```python
from build123d import *

# Parameters (mm, degrees)
SKETCH1_R           = 2.1
BOSS_EXTRUDE1_DEPTH = 1000


with BuildPart() as part:
    # Sketch1 → Boss-Extrude1 (new body)
    with BuildSketch(Plane(origin=(0, 0, 0), x_dir=(-1, 0, 0), z_dir=(0, 0, -1))):
        with BuildLine():
            Line((15.499339828, -8.2), (12.84, -8.2))
            Line((12.84, -8.2), (14.64, -10))
            Line((14.64, -10), (25.36, -10))
            Line((25.36, -10), (27.16, -8.2))
            Line((27.16, -8.2), (24.500660172, -8.2))
            Line((24.500660172, -8.2), (24.500660172, -6.56))
            Line((24.500660172, -6.56), (27.16, -3.900660172))
            Line((27.16, -3.900660172), (32.84, -3.900660172))
            Line((32.84, -3.900660172), (35.499339828, -6.56))
            Line((35.499339828, -6.56), (35.499339828, -8.2))
            Line((35.499339828, -8.2), (32.84, -8.2))
            Line((32.84, -8.2), (34.64, -10))
            Line((34.64, -10), (38, -10))
            ThreePointArc((38, -10), (39.414213562, -9.414213562), (40, -8))
            Line((40, -8), (40, -4.64))
            Line((40, -4.64), (38.2, -2.84))
            Line((38.2, -2.84), (38.2, -5.499339828))
            Line((38.2, -5.499339828), (36.56, -5.499339828))
            Line((36.56, -5.499339828), (33.900660172, -2.84))
            Line((33.900660172, -2.84), (33.900660172, 2.84))
            Line((33.900660172, 2.84), (36.56, 5.499339828))
            Line((36.56, 5.499339828), (38.2, 5.499339828))
            Line((38.2, 5.499339828), (38.2, 2.84))
            Line((38.2, 2.84), (40, 4.64))
            Line((40, 4.64), (40, 8))
            ThreePointArc((40, 8), (39.414213562, 9.414213562), (38, 10))
            Line((38, 10), (34.64, 10))
            Line((34.64, 10), (32.84, 8.2))
            Line((32.84, 8.2), (35.499339828, 8.2))
            Line((35.499339828, 8.2), (35.499339828, 6.56))
            Line((35.499339828, 6.56), (32.84, 3.900660172))
            Line((32.84, 3.900660172), (27.16, 3.900660172))
            Line((27.16, 3.900660172), (24.500660172, 6.56))
            Line((24.500660172, 6.56), (24.500660172, 8.2))
            Line((24.500660172, 8.2), (27.16, 8.2))
            Line((27.16, 8.2), (25.36, 10))
            Line((25.36, 10), (14.64, 10))
            Line((14.64, 10), (12.84, 8.2))
            Line((12.84, 8.2), (15.499339828, 8.2))
            Line((15.499339828, 8.2), (15.499339828, 6.56))
            Line((15.499339828, 6.56), (12.84, 3.900660172))
            Line((12.84, 3.900660172), (7.16, 3.900660172))
            Line((7.16, 3.900660172), (4.500660172, 6.56))
            Line((4.500660172, 6.56), (4.500660172, 8.2))
            Line((4.500660172, 8.2), (7.16, 8.2))
            Line((7.16, 8.2), (5.36, 10))
            Line((5.36, 10), (-5.36, 10))
            Line((-5.36, 10), (-7.16, 8.2))
            Line((-7.16, 8.2), (-4.500660172, 8.2))
            Line((-4.500660172, 8.2), (-4.500660172, 6.56))
            Line((-4.500660172, 6.56), (-7.16, 3.900660172))
            Line((-7.16, 3.900660172), (-12.84, 3.900660172))
            Line((-12.84, 3.900660172), (-15.499339828, 6.56))
            Line((-15.499339828, 6.56), (-15.499339828, 8.2))
            Line((-15.499339828, 8.2), (-12.84, 8.2))
            Line((-12.84, 8.2), (-14.64, 10))
            Line((-14.64, 10), (-25.36, 10))
            Line((-25.36, 10), (-27.16, 8.2))
            Line((-27.16, 8.2), (-24.500660172, 8.2))
            Line((-24.500660172, 8.2), (-24.500660172, 6.56))
            Line((-24.500660172, 6.56), (-27.16, 3.900660172))
            Line((-27.16, 3.900660172), (-32.84, 3.900660172))
            Line((-32.84, 3.900660172), (-35.499339828, 6.56))
            Line((-35.499339828, 6.56), (-35.499339828, 8.2))
            Line((-35.499339828, 8.2), (-32.84, 8.2))
            Line((-32.84, 8.2), (-34.64, 10))
            Line((-34.64, 10), (-38, 10))
            ThreePointArc((-38, 10), (-39.414213562, 9.414213562), (-40, 8))
            Line((-40, 8), (-40, 4.64))
            Line((-40, 4.64), (-38.2, 2.84))
            Line((-38.2, 2.84), (-38.2, 5.499339828))
            Line((-38.2, 5.499339828), (-36.56, 5.499339828))
            Line((-36.56, 5.499339828), (-33.900660172, 2.84))
            Line((-33.900660172, 2.84), (-33.900660172, -2.84))
            Line((-33.900660172, -2.84), (-36.56, -5.499339828))
            Line((-36.56, -5.499339828), (-38.2, -5.499339828))
            Line((-38.2, -5.499339828), (-38.2, -2.84))
            Line((-38.2, -2.84), (-40, -4.64))
            Line((-40, -4.64), (-40, -8))
            ThreePointArc((-40, -8), (-39.414213562, -9.414213562), (-38, -10))
            Line((-38, -10), (-34.64, -10))
            Line((-34.64, -10), (-32.84, -8.2))
            Line((-32.84, -8.2), (-35.499339828, -8.2))
            Line((-35.499339828, -8.2), (-35.499339828, -6.56))
            Line((-35.499339828, -6.56), (-32.84, -3.900660172))
            Line((-32.84, -3.900660172), (-27.16, -3.900660172))
            Line((-27.16, -3.900660172), (-24.500660172, -6.56))
            Line((-24.500660172, -6.56), (-24.500660172, -8.2))
            Line((-24.500660172, -8.2), (-27.16, -8.2))
            Line((-27.16, -8.2), (-25.36, -10))
            Line((-25.36, -10), (-14.64, -10))
            Line((-14.64, -10), (-12.84, -8.2))
            Line((-12.84, -8.2), (-15.499339828, -8.2))
            Line((-15.499339828, -8.2), (-15.499339828, -6.56))
            Line((-15.499339828, -6.56), (-12.84, -3.900660172))
            Line((-12.84, -3.900660172), (-7.16, -3.900660172))
            Line((-7.16, -3.900660172), (-4.500660172, -6.56))
            Line((-4.500660172, -6.56), (-4.500660172, -8.2))
            Line((-4.500660172, -8.2), (-7.16, -8.2))
            Line((-7.16, -8.2), (-5.36, -10))
            Line((-5.36, -10), (5.36, -10))
            Line((5.36, -10), (7.16, -8.2))
            Line((7.16, -8.2), (4.500660172, -8.2))
            Line((4.500660172, -8.2), (4.500660172, -6.56))
            Line((4.500660172, -6.56), (7.16, -3.900660172))
            Line((7.16, -3.900660172), (12.84, -3.900660172))
            Line((12.84, -3.900660172), (15.499339828, -6.56))
            Line((15.499339828, -6.56), (15.499339828, -8.2))
        make_face()
        with Locations(Location((10, 0, 0), (0, 0, 180))):
            Circle(SKETCH1_R, mode=Mode.SUBTRACT)
        with Locations(Location((30, 0, 0), (0, 0, 180))):
            Circle(SKETCH1_R, mode=Mode.SUBTRACT)
        with Locations(Location((-10, 0, 0), (0, 0, 180))):
            Circle(SKETCH1_R, mode=Mode.SUBTRACT)
        with Locations(Location((-30, 0, 0), (0, 0, 180))):
            Circle(SKETCH1_R, mode=Mode.SUBTRACT)
        Polygon((17.300660172, -6.24), (13.900660172, -2.84), (13.900660172, 2.84), (17.300660172, 6.24), (17.300660172, 8.2), (22.699339828, 8.2), (22.699339828, 6.24), (26.099339828, 2.84), (26.099339828, -2.84), (22.699339828, -6.24), (22.699339828, -8.2), (17.300660172, -8.2), align=None, mode=Mode.SUBTRACT)
        Polygon((2.699339828, 6.24), (6.099339828, 2.84), (6.099339828, -2.84), (2.699339828, -6.24), (2.699339828, -8.2), (-2.699339828, -8.2), (-2.699339828, -6.24), (-6.099339828, -2.84), (-6.099339828, 2.84), (-2.699339828, 6.24), (-2.699339828, 8.2), (2.699339828, 8.2), align=None, mode=Mode.SUBTRACT)
        Polygon((-13.900660172, -2.84), (-17.300660172, -6.24), (-17.300660172, -8.2), (-22.699339828, -8.2), (-22.699339828, -6.24), (-26.099339828, -2.84), (-26.099339828, 2.84), (-22.699339828, 6.24), (-22.699339828, 8.2), (-17.300660172, 8.2), (-17.300660172, 6.24), (-13.900660172, 2.84), align=None, mode=Mode.SUBTRACT)
    extrude(amount=-BOSS_EXTRUDE1_DEPTH)


solid = part.part
```
Input: part model. Units: mm. Frame: model coordinates. Give positions to 0.01 mm unless a question says otherwise; leave off trailing zeros. Return JSON: item names as keys, results as strings.
1) Contact query for flat-ended pins moving along their axis: pin 1 (3 mm diameter, centred on y = 0.5, z = 516, fed in from +X); pin 2 (6 mm diameter, centred on x = -31, z = 520.5, fed in from +Y); pin 3 (1.7 mm diameter, centred on x = 29.5, z = 351.5, fed in from -Y). Output: stop coordinate, or through.
Taken from the geometry:
{"pin 1": "stops at x = 33.9", "pin 2": "stops at y = 9.36", "pin 3": "stops at y = -3.9"}
2) Line query: L1, parallel to Y at x = 35, z = 342; L2, parallel to X at y = 3, z = 201.5; L3, parallel to Y at x = 30, z = 336.5. Output: solid intervals per line, ascending. Write a range as [from, to].
Taken from the geometry:
{"L1": "y = [-10, -8.2], [-6.06, -3.94], [3.94, 6.06], [8.2, 10]", "L2": "x = [-38.36, -38.2], [-34.06, -25.94], [-14.06, -5.94], [5.94, 14.06], [25.94, 34.06], [38.2, 38.36]", "L3": "y = [-3.9, -2.1], [2.1, 3.9]"}
3) Section query A-A on z = 389. Count the separate pieces of the cut face and the enclosed holes in it, and give its area (3 significant figures).
Taken from the geometry:
{"separate pieces": "1", "enclosed holes": "7", "area": "554 mm2"}
